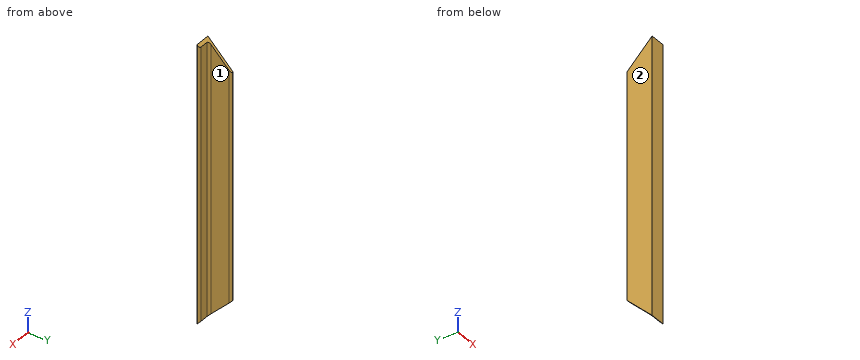
Autodesk Inventor part; units mm, degrees
ref_plane "Start Plane" through (0, 0, -24.2929) normal (0, 0, 1) x (1, 0, 0)
ref_plane "End Plane" through (0, 0, 524.2929) normal (0, 0, 1) x (1, 0, 0)
ref_plane "Work Plane11" through (7.59, -17.6536, 524.6464) normal (0, 0.7071, 0.7071) x (1, 0, 0)
ref_plane "Start Plane" through (0, 0, -24.2929) normal (0, 0, 1) x (1, 0, 0)
ref_plane "End Plane" through (0, 0, 524.2929) normal (0, 0, 1) x (1, 0, 0)
sketch "Sketch" plane through (0, 0, 0) normal (0, 0, 1) x (1, 0, 0)
  line L0 (-2.41, 28.7) -> (-2.41, -7.3)
  line L1 (-7.41, 32.7) -> (-6.41, 32.7)
  line L2 (-7.41, -17.3) -> (-7.41, 32.7)
  line L3 (22.59, -17.3) -> (-7.41, -17.3)
  line L4 (22.59, -16.3) -> (22.59, -17.3)
  line L5 (2.59, -12.3) -> (18.59, -12.3)
  arc A0 (-2.41, -7.3) -> (2.59, -12.3) centre (2.59, -7.3) ccw
  arc A1 (-2.41, 28.7) -> (-6.41, 32.7) centre (-6.41, 28.7) ccw
  arc A2 (22.59, -16.3) -> (18.59, -12.3) centre (18.59, -16.3) ccw
  line L6 (0, 43.6941) -> (0, -27.4657) construction
  line L7 (-13.5757, 0) -> (29.5841, 0) construction
  point P0 (-2.41, 32.7)
  point P1 (-2.41, -12.3)
  point P2 (22.59, -12.3)
  dimension "d4" = 30
  dimension "d6" = 50
  dimension "d8" = 5
  dimension "d10" = 5
  dimension "d17" = 5
  dimension "d18" = 4
  dimension "d19" = 17.3
  dimension "d20" = 7.41
extrude "Body" add sketch "Sketch" along normal up to surface (548.5858 mm away) from surface at -24.2929
sketch "Sketch3" plane through (0, 0, 0) normal (0, 0, 1) x (1, 0, 0)
  line L0 (0, 0) -> (10, 0)
ref_plane "Work Plane10" through (0, 0, 0) normal (0, -1, 0) x (1, 0, 0)
sketch "Sketch4" plane through (0, 0, 0) normal (0, -1, 0) x (1, 0, 0)
  line L0 (-2, -24.2929) -> (12, -24.2929)
  line L1 (-2, 524.2929) -> (12, 524.2929)
  dimension "d24" = 548.5858
ref_plane "Work Plane11" through (7.59, -17.6536, 524.6464) normal (0, 0.7071, 0.7071) x (1, 0, 0)
split "Split1" plane through (7.59, -17.6536, 524.6464) removes the side toward (0, 0.7071, 0.7071)
ref_plane "Work Plane12" through (7.59, -17.6536, -24.6464) normal (0, 0.7071, -0.7071) x (1, 0, 0)
split "Split2" plane through (7.59, -17.6536, -24.6464) removes the side toward (0, 0.7071, -0.7071)
equation "\"d4\" = b"
equation "\"d6\" = ParH"
equation "\"d17\" = R"
equation "\"d18\" = R1"
equation "\"d19\" = ex"
equation "\"d20\" = ey"
equation "\"d11\" = G_L"
equation "\"b\" = 30"
equation "\"ParT\" = 5"
equation "\"R1\" = 4"
equation "\"G_L\" = d24"
equation "\"ParH\" = 50"
equation "\"R\" = 5"
equation "\"ey\" = 7.41"
equation "\"ex\" = 17.3"
equation "\"G_OFFSET_START\" = 24.29289"
equation "\"G_OFFSET_END\" = 24.29289"
equation "\"d21\" = -G_OFFSET_START"
equation "\"d22\" = G_OFFSET_END + B_L"
properties part number "ISO 657-2 - 50x 30x 5-548.59" material "Steel, Mild"
Part model, mm, in its own coordinate system. Face numbers are marked on the shaded views. A direction names the side the tool comes from. Coordinates: 2 decimals unless noted, no trailing zeros. Write each loop counter-clockwise with the first axis right and the second up, starting at its lowest first coordinate (ties: lowest second). Pieces come first, ordered by that corner, then holes.
Item 1: Slice it at A-A (z = 74.5). Write the cut outline in (x, y).
Item 2: Slice it at C-C (y = 21.5). Write the cut outline in (x, z), and give its area (3 significant figures).
Item 3: Probe line 1 (X direction, y = 25.5, z = 162); line 2 (Y direction, x = 4.75, z = 491.5); line 3 (Y direction, x = -5.75, z = 240). List the from-to ranges inside material, lowest first.
Item 4: Slice it at B-B (x = 7.5). Write the cut outline in (y, z).
Item 5: Pin check, flat tips, straight feed: pin 1 (4 mm diameter, centred on x = -1, y = -4.5, fed in from +Z); pin 2 (17.5 mm diameter, centred on x = 9.5, z = 258.5, fed in from +Y); pin 3 (8 mm diameter, centred on x = 3.5, y = 19, fed in from +Z); pin 4 (11 mm diameter, centred on y = 2, z = 208.5, fed in from +X). Stop position of each tip, or through.
Item 6: Which spindle directions (+Z, -Z, +X, -X, +Y, -Y) get a long thin tool onto all of the face, cutting with end or side? Do the marked faces 1 and 2. Say none if no direction does.
Results found:
1. outline: (-7.41, -17.3) - (22.59, -17.3) - (22.59, -16.3) arc R4 ccw to (18.59, -12.3) - (2.59, -12.3) arc R5 cw to (-2.41, -7.3) - (-2.41, 28.7) arc R4 ccw to (-6.41, 32.7) - (-7.41, 32.7) - close
2. outline: (-7.41, 14.51) - (-2.41, 14.51) - (-2.41, 485.49) - (-7.41, 485.49) - close
2. area: 2,350 mm2
3. line 1: x = -7.41 to -2.41
3. line 2: y = -17.3 to -12.3
3. line 3: y = -17.3 to 32.65
4. outline: (-17.3, -24.29) - (-12.3, -19.29) - (-12.3, 519.29) - (-17.3, 524.29) - close
5. pin 1: stops at z = 512.91
5. pin 2: stops at y = -11.95
5. pin 3: passes through
5. pin 4: stops at x = -2.41
6. face 1: +Z, -Z, +X, +Y
6. face 2: +Z, -Z, -X, +Y, -Y
